from build123d import *

# Parameters (mm, degrees)
PAD_DEPTH            = 20
PAD001_DEPTH         = 20
PAD002_DEPTH         = 12
SKETCH004_R          = 8
POCKET001_DEPTH      = 20.001
POCKET001_DEPTH_BACK = -20.001
SKETCH005_R          = 8
POCKET002_DEPTH      = 0.001
POCKET002_DEPTH_BACK = -60.001


with BuildPart() as part:
    # Sketch → Pad (new body, symmetric)
    with BuildSketch(Plane.XZ):
        with BuildLine():
            Line((0, 60), (0, 0))
            Line((0, 0), (12, 0))
            Line((12, 0), (12, 20))
            ThreePointArc((22, 30), (14.928932, 27.071068), (12, 20))
            Line((60, 30), (22, 30))
            Line((60, 30), (60, 42))
            Line((45, 42), (60, 42))
            ThreePointArc((40, 47), (41.464466, 43.464466), (45, 42))
            Line((40, 60), (40, 47))
            Line((40, 60), (0, 60))
        make_face()
    extrude(amount=PAD_DEPTH, both=True)

    # Sketch001 → Pad001 (join, symmetric)
    with BuildSketch(Plane.XZ):
        with BuildLine():
            ThreePointArc((40, 60), (20, 80), (0, 60))
            Line((40, 60), (0, 60))
        make_face()
    extrude(amount=PAD001_DEPTH, both=True)

    # Sketch002 → Pad002 (join)
    with BuildSketch(Plane.YZ):
        with BuildLine():
            ThreePointArc((-20, 0), (0, -20), (20, 0))
            Line((20, 0), (-20, 0))
        make_face()
    extrude(amount=PAD002_DEPTH)

    # Sketch004 → Pocket001 (cut, two sides)
    with BuildSketch(Plane.XZ) as pocket001_sk:
        with Locations((20, 60)):
            Circle(SKETCH004_R)
    extrude(amount=-POCKET001_DEPTH, mode=Mode.SUBTRACT)
    extrude(pocket001_sk.sketch, amount=-POCKET001_DEPTH_BACK, mode=Mode.SUBTRACT)

    # Sketch005 → Pocket002 (cut, two sides)
    with BuildSketch(Plane.YZ) as pocket002_sk:
        Circle(SKETCH005_R)
    extrude(amount=-POCKET002_DEPTH, mode=Mode.SUBTRACT)
    extrude(pocket002_sk.sketch, amount=-POCKET002_DEPTH_BACK, mode=Mode.SUBTRACT)


solid = part.part
For this review, take the finished solid that the model builds, in its own axes (mm). A direction names the side the tool comes from. Give positions to 0.01 mm unless a question says otherwise; leave off trailing zeros. Loops run counter-clockwise (first coordinate to the right, second up) from the corner with the lowest first, then second, coordinate; pieces in that order, holes last. Notation, with made-up numbers: M 70.5,-36.75 L 74.5,-36.75 A10 cw 74.5,-30.75 Z; hole C -26.75,75 d2. An arc over 180 degrees is marked long. Answer as a JSON object with one key per item and string values. Group by question number.
Q1. Insertion check: P1, Ø1.5, axis at y = -8.5, z = -3.5, coming from the -X side; P2, Ø10, axis at x = 36.5, y = -12.5, coming from the -Z side; P3, Ø1, axis at x = 13, y = 15, coming from the +Z side; P4, Ø4, axis at x = 9, y = -14.5, coming from the -Z side. Each pin has a flat end and moves straight along its axis. Give the tip position at first contact, or say it passes through.
Q2. Add section B-B on x = 20. Give the boundary of the cut face in (y, z).
Q3. For probe 1 along X at (y, z) = (-14, 60); probe 2 along Y at (x, z) = (7, 0); probe 3 along X at (y, z) = (16, 5), list the stretches that pass through material, from the lowest coordinate up. Write a range as [from, to].
Q4. Add section A-A on y = 2. Give the boundary of the cut face in (x, z), and give its area (3 significant figures).
Q5. Mouldability with a two-part tool opening along Z and no side actions: class faces 1 (the cylindrical face through (41, 0, 44)), 2 (the flat face through (60, 0, 36)), 3 (the cylindrical face through (5.92, -1.73, -7.81)) as +Z half, -Z half, draft (parallel to the pull), parting line (faces both ways), or undercut.
Q6. Add section D-D on z = 16. Give the boundary of the cut face in (x, y).
Q7. Add section C-C on y = -14. Give the boundary of the cut face in (x, z), and give its area (3 significant figures).
Q8. Tool access review of faces 4 (the cylindrical face through (20, 0, 80)), 5 (the flat face through (12, 0, 9)), 6 (the flat face through (52, 0, 42)): name each direction out of +Z, -Z, +X, -X, +Y, -Y from which nothing blocks a thin tool from reaching the whole face with its end or side.
Checked values:
{
 "1": {"P1": "x = 0", "P2": "z = 30", "P3": "z = 78.91", "P4": "z = -15.61"},
 "2": {"outline": "M -20,29.8 L 20,29.8 L 20,52 L -20,52 Z; M -20,68 L 20,68 L 20,80 L -20,80 Z"},
 "3": {"probe 1": "[0, 12], [28, 40]", "probe 2": "[-20, -8], [8, 20]", "probe 3": "[0, 12]"},
 "4": {"outline": "M 0,-19.9 L 12,-19.9 L 12,-7.75 L 0,-7.75 Z; M 0,7.75 L 12,7.75 L 12,20 A10 cw 22,30 L 60,30 L 60,42 L 45,42 A5 cw 40,47 L 40,60 A20 ccw 0,60 Z; hole C 20,60 d16", "area": "2,310 mm²"},
 "5": {"face 1": "+Z half", "face 2": "draft", "face 3": "undercut"},
 "6": {"outline": "M 0,-20 L 12,-20 L 12,20 L 0,20 Z"},
 "7": {"outline": "M 0,-14.28 L 12,-14.28 L 12,20 A10 cw 22,30 L 60,30 L 60,42 L 45,42 A5 cw 40,47 L 40,60 A20 ccw 0,60 Z; hole C 20,60 d16", "area": "2,430 mm²"},
 "8": {"face 4": "+Z, +Y, -Y", "face 5": "-Z, +X, +Y, -Y", "face 6": "+Z, +X, +Y, -Y"}
}
